Check sheet for the modelled part. Datum: model origin and axes. Units: mm. Face numbers are marked on the shaded views. A direction names the side the tool comes from. Coordinates: 2 decimals unless noted, no trailing zeros. Order: outer loops, then holes, each group sorted by start corner. A loop starts at its lowest first (then second) coordinate and runs counter-clockwise, first axis right, second up.
1. Cross-section at D-D (y = 140). Enter the section's corners in (x, z).
2. Thickness scan on line 1 (Y direction, x = -10.5, z = -3.3); line 2 (X direction, y = 23, z = -3); line 3 (Z direction, x = 55.5, y = 217.5). Record the ranges inside material, lowest first.
3. Cross-section at B-B (z = 19). Enter the section's corners in (x, y).
4. Gauge pin test, flat ends, axial feed: pin 1 Ø4 at (x, y) = (-10.5, 7) entering from +Z; pin 2 Ø9 at (x, z) = (-21, 17) entering from -Y; pin 3 Ø6.5 at (x, y) = (-20.5, 21.5) entering from +Z. Record the tip position at first contact, or that the pin passes through.
5. Cross-section at A-A (y = 38.5). Enter the section's corners in (x, z).
6. Set-up check for the marked faces 1, 2 and 3: record each of +Z, -Z, +X, -X, +Y, -Y from which the full face is reachable in a straight line by a thin tool's end or side.
7. Cross-section at C-C (x = 8). Enter the section's corners in (y, z), then the cut area to 3 significant figures.
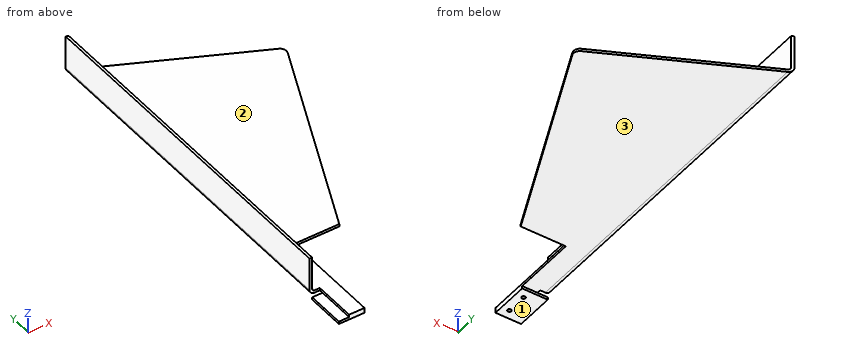
```python
from build123d import *

# Parameters (mm, degrees)
F1_DEPTH = 400
F2_W     = 221.745663
F2_H     = 423.016819
F3_DEPTH = 50
F4_R     = 1.45
F5_DEPTH = 25
F6_W     = 8
F6_H     = 30
F6_W_2   = 12
F6_R     = 1.45
F7_DEPTH = 2


with BuildPart() as f1:
    # F0 (on Front) → F1 (new body)
    with BuildSketch(Plane.XZ):
        with BuildLine():
            Line((-22.5, 2), (-22.5, 28))
            Line((-22.5, 28), (-24.5, 28))
            Line((-24.5, 28), (-24.5, 2))
            ThreePointArc((-24.5, 2), (-23.328427, -0.828427), (-20.5, -2))
            Line((-20.5, -2), (125.5, -2))
            Line((125.5, -2), (125.5, 0))
            Line((125.5, 0), (-20.5, 0))
            ThreePointArc((-20.5, 0), (-21.914214, 0.585786), (-22.5, 2))
        make_face()
    extrude(amount=-F1_DEPTH)

    # F2 (on Top) → F3 (cut, symmetric)
    with BuildSketch(Plane.XY):
        with Locations((54.499505, 198.406644)):
            Rectangle(F2_W, F2_H)
        with BuildLine():
            Line((-24.5, 33), (-24.5, 307.38047))
            Line((-24.5, 307.38047), (100.260685, 247.214851))
            ThreePointArc((100.260685, 247.214851), (102.783459, 244.43172), (102.656531, 240.67751))
            Line((102.656531, 240.67751), (30.705116, 79.071984))
            Line((30.705116, 79.071984), (-4.5, 79.071984))
            Line((-4.5, 79.071984), (-4.5, 0))
            Line((-4.5, 0), (-16.5, 0))
            Line((-16.5, 0), (-16.5, 33))
            Line((-16.5, 33), (-24.5, 33))
        make_face(mode=Mode.SUBTRACT)
    extrude(amount=F3_DEPTH, both=True, mode=Mode.SUBTRACT)

    # F4 (on face) → F5 (cut)
    with BuildSketch(Plane(origin=(0, 0, -2), x_dir=(1, 0, 0), z_dir=(0, 0, -1))):
        with Locations((-18.5, -7)):
            Circle(F4_R)
        with Locations((-18.5, -23)):
            Circle(F4_R)
    extrude(amount=-F5_DEPTH, mode=Mode.SUBTRACT)

    # F6 (on face) → F7 (join)
    with BuildSketch(Plane(origin=(0, 0, -2), x_dir=(1, 0, 0), z_dir=(0, 0, -1))):
        with Locations((-20.5, -15)):
            Rectangle(F6_W, F6_H)
        with Locations((-10.5, -15)):
            Rectangle(F6_W_2, F6_H)
        with Locations((-10.5, -23)):
            Circle(F6_R, mode=Mode.SUBTRACT)
        with Locations((-10.5, -7)):
            Circle(F6_R, mode=Mode.SUBTRACT)
    extrude(amount=F7_DEPTH)


solid = f1.part
```
Data:
1. outline: (-24.5, 2) arc R4 ccw to (-20.5, -2) - (57.83, -2) - (57.83, 0) - (-20.5, 0) arc R2 cw to (-22.5, 2) - (-22.5, 28) - (-24.5, 28) - close
2. line 1: y = 0 to 5.55, 8.45 to 21.55, 24.45 to 30
2. line 2: x = -24.5 to -11.95, -9.05 to -4.5
2. line 3: z = -2 to 0
3. outline: (-24.5, 33) - (-22.5, 33) - (-22.5, 306.42) - (-24.5, 307.38) - close
4. pin 1: stops at z = 0
4. pin 2: stops at y = 33
4. pin 3: stops at z = -2
5. outline: (-24.5, 2) arc R4 ccw to (-20.5, -2) - (-4.5, -2) - (-4.5, 0) - (-20.5, 0) arc R2 cw to (-22.5, 2) - (-22.5, 28) - (-24.5, 28) - close
6. face 1: -Z, +X, -X, +Y, -Y
6. face 2: +Z, +X, +Y, -Y
6. face 3: -Z, +X, -X, +Y
7. outline: (79.07, -2) - (291.71, -2) - (291.71, 0) - (79.07, 0) - close
7. area: 425 mm2
